Input: dimensioned drawing with shaded views. Units: mm. Origin: part minimum x, y, z. Round coordinates to 2 decimals unless told otherwise and drop trailing zeros. Loops run counter-clockwise (first coordinate to the right, second up) from the corner with the lowest first, then second, coordinate; pieces in that order, holes last. Notation, with made-up numbers: M 35.5,-7.5 L 77.5,-7.5 A23 ccw 77.5,19.5 Z; hole C 79,67 d8. An arc over 180 degrees is marked long. Write each question's results on one line, items separated by ' | '. Start each with the question number.
1. Contact query for a flat-ended pin moving along its axis: pin 1 Ø10 at (x, y) = (65, 55.5) entering from -Z. Output: stop coordinate, or through.
2. Section B-B on y = 108.5. Output: boundary loops of the cut face in (x, z).
3. Section A-A on x = 67.5. Output: boundary loops of the cut face in (y, z), and give its area (3 significant figures).
4. Ray query, line 1 (X direction, y = 21.5, z = 1); line 2 (Y direction, x = 67.5, z = 0.8). Return the intervals inside material, ascending.
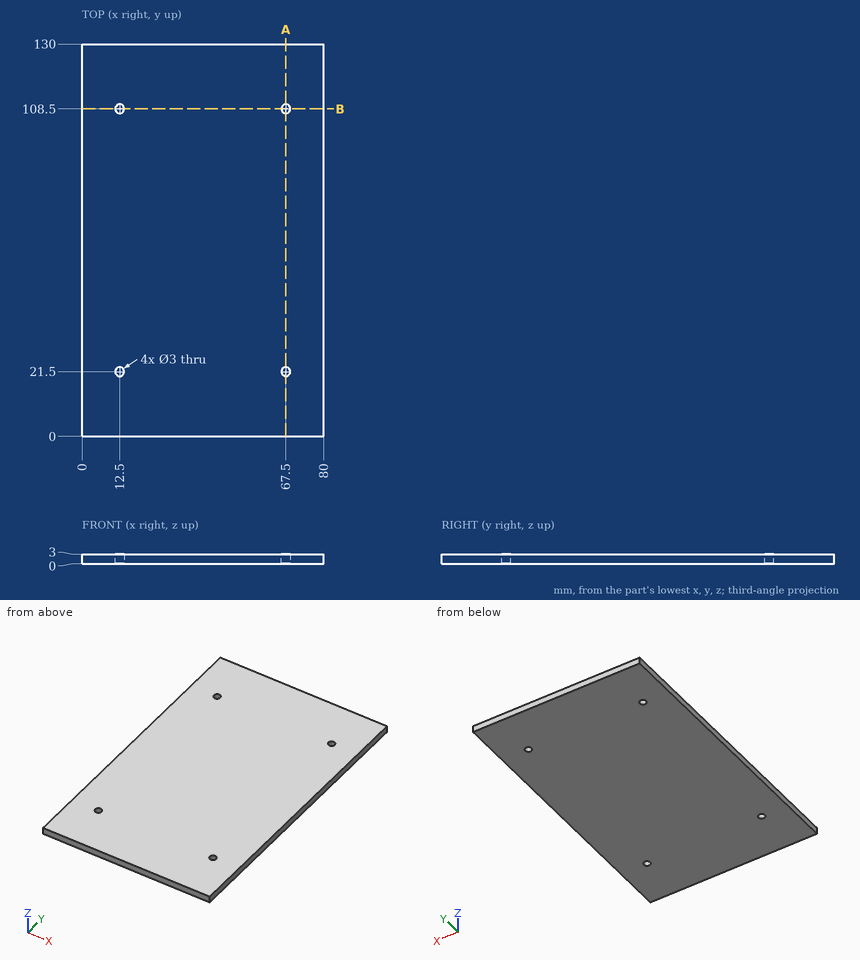
Taken from the geometry:
1) pin 1: z = 0
2) outline: M 0,0 L 11,0 L 11,3 L 0,3 Z; M 14,0 L 66,0 L 66,3 L 14,3 Z; M 69,0 L 80,0 L 80,3 L 69,3 Z
3) outline: M 0,0 L 20,0 L 20,3 L 0,3 Z; M 23,0 L 107,0 L 107,3 L 23,3 Z; M 110,0 L 130,0 L 130,3 L 110,3 Z | area: 372 mm^2
4) line 1: 0 to 11, 14 to 66, 69 to 80 | line 2: 0 to 20, 23 to 107, 110 to 130
